Source: CAD feature listing. Evaluate the final solid. Frame: model axes, mm. A direction names the side the tool comes from. Give positions to 0.01 mm unless a question says otherwise; leave off trailing zeros. Order: outer loops, then holes, each group sorted by start corner. A loop starts at its lowest first (then second) coordinate and runs counter-clockwise, first axis right, second up.
1) Material intervals for line 1 (X direction, y = 5, z = -32.5); line 2 (X direction, y = 4.75, z = -55); line 3 (X direction, y = 3.75, z = 25), sorted ascending.
2) Section B-B, the plane x = -25. Return loops of the section in (y, z).
3) Section C-C, the plane y = 4.5. Give the number of separate pieces and of enclosed holes in the cut face, plus the area to 3 significant figures.
4) Draft query along X for faces 3 (the face through (-30.15, 3.45, -79.42)), 4 (the face through (-82.129, 3.451, 82.518)), 5 (the face through (-29.596, 3.451, -19.428)), 6 (the face through (82.129, 3.451, -82.518)). Return one class per face: released by +X, released by -X, zero draft, split by the parting line, or undercut.
5) First-contact query: P1, Ø25, axis at x = 3.5, z = -76.5, coming from the -Y side; P2, Ø1.6, axis at y = 0.5, z = -87.5, coming from the -X side; P3, Ø5, axis at x = 14.8, z = -92.68, coming from the -Y side; P4, Ø1, axis at y = 1.5, z = -83.5, coming from the +X side. Flat tips, straight axial feed; report the tip coordinate or a pass-through.
6) Section D-D, the plane x = 37.5. Return loops of the section in (y, z).
7) Section A-A, the plane x = 85. Return loops of the section in (y, z), plus the area to 3 significant figures.
8) Access query for faces 1 (the face through (17.371, 3, -50)), 2 (the face through (1, 3, 100)). Directions: +Z, -Z, +X, -X, +Y, -Y. A direction counts if a zero-diameter tool reaches every point of the face in a straight line with its end or side. Return the directions, or none.
```python
from build123d import *

# Parameters (mm, degrees)
SKETCH1_R           = 6
BOSS_EXTRUDE2_DEPTH = 7
SKETCH2_R           = 2
CUT_EXTRUDE1_DEPTH  = 142.594491418
SKETCH3_R           = 2
CUT_EXTRUDE3_DEPTH  = 142.594491418
SKETCH4_R           = 2
CUT_EXTRUDE4_DEPTH  = 142.594491418
SKETCH5_W           = 36
SKETCH5_H           = 31
CUT_EXTRUDE7_DEPTH  = 2


with BuildPart() as part:
    # Sketch1 → Boss-Extrude2 (new body)
    with BuildSketch(Plane(origin=(0, 0, 0), x_dir=(1, 0, 0), z_dir=(0, 1, 0))):
        with BuildLine():
            Line((-75, 100), (75, 100))
            ThreePointArc((75, 100), (82.32233047, 82.32233047), (100, 75))
            Line((100, 75), (100, -75))
            ThreePointArc((100, -75), (82.32233047, -82.32233047), (75, -100))
            Line((75, -100), (-75, -100))
            ThreePointArc((-75, -100), (-82.32233047, -82.32233047), (-100, -75))
            Line((-100, -75), (-100, 75))
            ThreePointArc((-100, 75), (-82.32233047, 82.32233047), (-75, 100))
        make_face()
        with Locations(Location((-85, 55, 0), (0, 0, 270))):
            Circle(SKETCH1_R, mode=Mode.SUBTRACT)
        with Locations(Location((85, 55, 0), (0, 0, 270))):
            Circle(SKETCH1_R, mode=Mode.SUBTRACT)
        with Locations(Location((25, -85, 0), (0, 0, 270))):
            Circle(SKETCH1_R, mode=Mode.SUBTRACT)
        with Locations(Location((-25, -85, 0), (0, 0, 270))):
            Circle(SKETCH1_R, mode=Mode.SUBTRACT)
        with BuildLine():
            Line((-17.370892019, 66.924882629), (-17.370892019, 31.924882629))
            ThreePointArc((-17.370892019, 31.924882629), (-29.870892019, 19.424882629), (-42.370892019, 31.924882629))
            Line((-42.370892019, 31.924882629), (-42.370892019, 66.924882629))
            ThreePointArc((-42.370892019, 66.924882629), (-29.870892019, 79.424882629), (-17.370892019, 66.924882629))
        make_face(mode=Mode.SUBTRACT)
        with BuildLine():
            Line((17.370892019, 66.924882629), (17.370892019, 31.924882629))
            ThreePointArc((17.370892019, 31.924882629), (29.870892019, 19.424882629), (42.370892019, 31.924882629))
            Line((42.370892019, 31.924882629), (42.370892019, 66.924882629))
            ThreePointArc((42.370892019, 66.924882629), (29.870892019, 79.424882629), (17.370892019, 66.924882629))
        make_face(mode=Mode.SUBTRACT)
        with BuildLine():
            ThreePointArc((-47.767999672, -52.36655043), (-0.196924647, -73.88254423), (48.43804341, -54.893467096))
            ThreePointArc((48.43804341, -54.893467096), (48.645377153, -40.752851384), (34.504761441, -40.545517641))
            ThreePointArc((34.504761441, -40.545517641), (0.328207745, -53.889439519), (-33.100731657, -38.769813727))
            ThreePointArc((-33.100731657, -38.769813727), (-47.232734016, -38.234548071), (-47.767999672, -52.36655043))
        make_face(mode=Mode.SUBTRACT)
    extrude(amount=BOSS_EXTRUDE2_DEPTH)

    # Sketch2 → Cut-Extrude1 (cut, through all)
    with BuildSketch(Plane(origin=(0, 7, 0), x_dir=(1, 0, 0), z_dir=(0, 1, 0))):
        with Locations(Location((-91, -25, 0), (0, 0, 270))):
            Circle(SKETCH2_R)
        with Locations(Location((0, 80, 0), (0, 0, 270))):
            Circle(SKETCH2_R)
        with Locations(Location((91, -25, 0), (0, 0, 270))):
            Circle(SKETCH2_R)
    extrude(amount=-CUT_EXTRUDE1_DEPTH, mode=Mode.SUBTRACT)

    # Sketch3 → Cut-Extrude3 (cut, through all)
    with BuildSketch(Plane(origin=(0, 7, 0), x_dir=(1, 0, 0), z_dir=(0, 1, 0))):
        with Locations(Location((-91, -35, 0), (0, 0, 270))):
            Circle(SKETCH3_R)
        with Locations(Location((91, -35, 0), (0, 0, 270))):
            Circle(SKETCH3_R)
    extrude(amount=-CUT_EXTRUDE3_DEPTH, mode=Mode.SUBTRACT)

    # Sketch4 → Cut-Extrude4 (cut, through all)
    with BuildSketch(Plane(origin=(0, 7, 0), x_dir=(1, 0, 0), z_dir=(0, 1, 0))):
        with Locations(Location((-14.796, 67.317, 0), (0, 0, 270))):
            Circle(SKETCH4_R)
        with Locations(Location((-14.796, 92.683, 0), (0, 0, 270))):
            Circle(SKETCH4_R)
        with Locations(Location((14.796833333, 92.683, 0), (0, 0, 270))):
            Circle(SKETCH4_R)
        with Locations(Location((14.796833333, 67.317, 0), (0, 0, 270))):
            Circle(SKETCH4_R)
    extrude(amount=-CUT_EXTRUDE4_DEPTH, mode=Mode.SUBTRACT)

    # Sketch5 → Cut-Extrude7 (cut)
    with BuildSketch(Plane.XZ):
        with Locations((0, -80)):
            Rectangle(SKETCH5_W, SKETCH5_H)
    extrude(amount=-CUT_EXTRUDE7_DEPTH, mode=Mode.SUBTRACT)


solid = part.part
```
From the geometry:
1. line 1: x = -100 to -42.37, -17.37 to 17.37, 42.37 to 100
1. line 2: x = -100 to -91, -79 to -42.37, -17.37 to 17.37, 42.37 to 79, 91 to 100
1. line 3: x = -100 to -93, -89 to 89, 93 to 100
2. outline: (0, -100) - (7, -100) - (7, -78.44) - (0, -78.44) - close; (0, -20.41) - (7, -20.41) - (7, 45.73) - (0, 45.73) - close; (0, 68.44) - (7, 68.44) - (7, 79) - (0, 79) - close; (0, 91) - (7, 91) - (7, 100) - (0, 100) - close
3. separate pieces: 1
3. enclosed holes: 16
3. area: 32,600 mm2
4. face 3: undercut
4. face 4: released by -X
4. face 5: undercut
4. face 6: released by +X
5. P1: stops at y = 0
5. P2: stops at x = -78.83
5. P3: stops at y = 2
5. P4: stops at x = 81.67
6. outline: (0, -100) - (7, -100) - (7, -76.83) - (0, -76.83) - close; (0, -22.02) - (7, -22.02) - (7, 38.54) - (0, 38.54) - close; (0, 63.51) - (7, 63.51) - (7, 100) - (0, 100) - close
7. outline: (0, -80) - (7, -80) - (7, -61) - (0, -61) - close; (0, -49) - (7, -49) - (7, 80) - (0, 80) - close
7. area: 1,040 mm2
8. face 1: +Y, -Y
8. face 2: +Z, +X, -X, +Y, -Y
